Drawing for the job (mm, zero at the part's lowest x, y, z). Round coordinates to 2 decimals unless told otherwise and drop trailing zeros. Write each loop counter-clockwise with the first axis right and the second up, starting at its lowest first coordinate (ties: lowest second). Pieces come first, ordered by that corner, then holes. Notation, with made-up numbers: (-7, -9.75) -> (28, -9.75) arc R22 cw to (28, 21.25) -> close; hole circle Ø9 at (69, 40). An arc over 180 degrees is marked (long way). Answer in a Markdown table with one row per item. Add a question column.
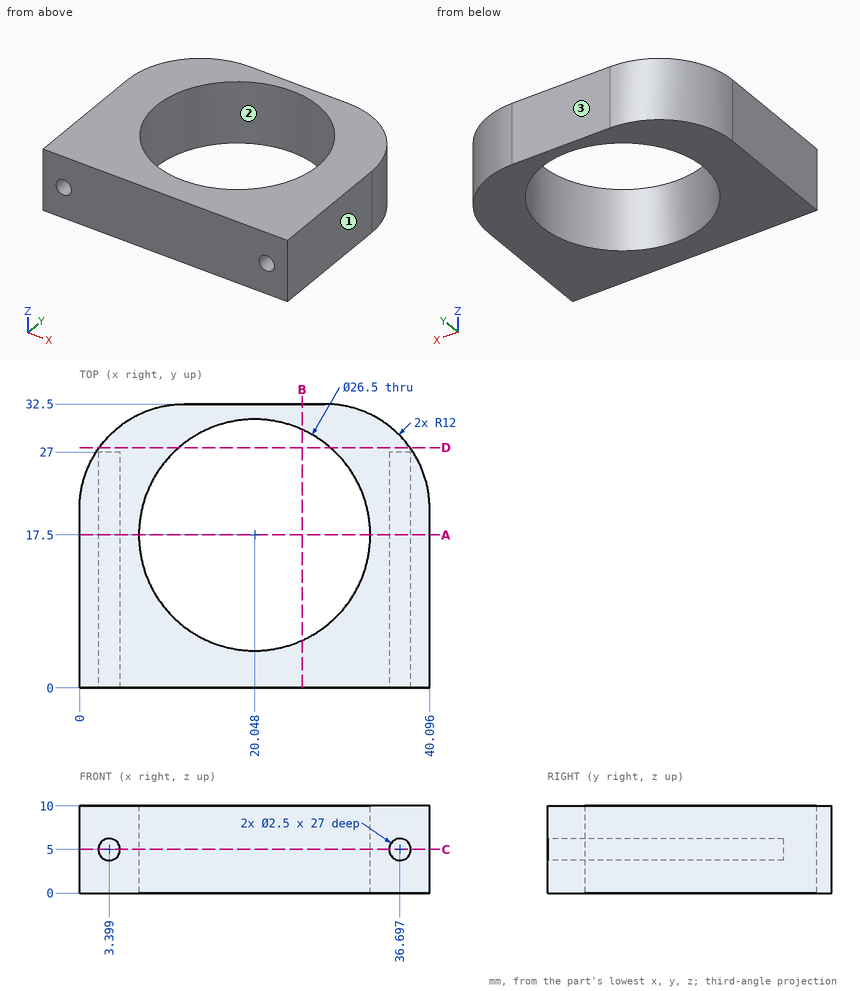
(1) Saw through at D-D (y = 27.5). List the corners of the cut face in (x, z).
(2) Probe line 1 along X through (y, z) = (13, 4.75); line 2 along Y through (x, z) = (29, 6); line 3 along Y through (x, z) = (23, 1.5). List the from-to ranges inside material, lowest first.
(3) Drop flat-ended pins along their axis: P1, Ø3, axis at x = 3.399, z = 5, coming from the +Y side; P2, Ø5, axis at x = 35, z = 2.5, coming from the +Y side; P3, Ø2, axis at x = 36.697, z = 5, coming from the -Y side. Give the stop position or say it passes through.
(4) Saw through at C-C (z = 5). List the corners of the cut face in (x, y).
(5) Mould opens along X. For the marked faces 1, 2 and 3 say: pulls with the +X half, pulls with the -X half, needs draft (parallel to the pull), parting line crosses it, or undercut.
(6) Saw through at B-B (x = 25.5). List the corners of the cut face in (y, z).
(7) Saw through at A-A (y = 17.5). List the corners of the cut face in (x, z), plus the area to 3 significant figures.
Answer sheet:
| question | item | result |
|---|---|---|
| 1 | outline | (2.25, 0) -> (11.36, 0) -> (11.36, 10) -> (2.25, 10) -> close; (28.74, 0) -> (37.84, 0) -> (37.84, 10) -> (28.74, 10) -> close |
| 2 | line 1 | x = 0 to 2.17, 4.62 to 7.59, 32.51 to 35.47, 37.92 to 40.1 |
| 2 | line 2 | y = 0 to 7.73, 27.27 to 32.47 |
| 2 | line 3 | y = 0 to 4.58, 30.42 to 32.5 |
| 3 | P1 | stops at y = 30.17 |
| 3 | P2 | stops at y = 31.66 |
| 3 | P3 | stops at y = 27 |
| 4 | outline | (0, 0) -> (2.15, 0) -> (2.15, 27) -> (4.65, 27) -> (4.65, 0) -> (35.45, 0) -> (35.45, 27) -> (37.95, 27) -> (37.95, 0) -> (40.1, 0) -> (40.1, 20.5) arc R12 ccw to (28.1, 32.5) -> (12, 32.5) arc R12 ccw to (0, 20.5) -> close; hole circle Ø26.5 at (20.05, 17.5) |
| 5 | face 1 | pulls with the +X half |
| 5 | face 2 | undercut |
| 5 | face 3 | needs draft |
| 6 | outline | (0, 0) -> (5.42, 0) -> (5.42, 10) -> (0, 10) -> close; (29.58, 0) -> (32.5, 0) -> (32.5, 10) -> (29.58, 10) -> close |
| 7 | outline | (0, 0) -> (6.8, 0) -> (6.8, 10) -> (0, 10) -> close; (33.3, 0) -> (40.1, 0) -> (40.1, 10) -> (33.3, 10) -> close; hole circle Ø2.5 at (3.4, 5); hole circle Ø2.5 at (36.7, 5) |
| 7 | area | 126 mm² |
